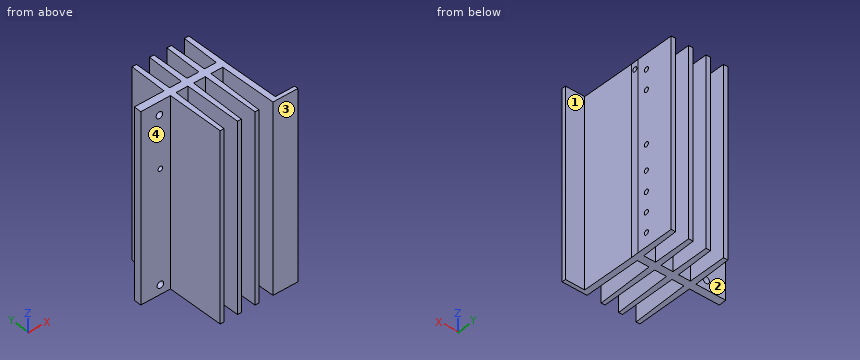
```python
from build123d import *

# Parameters (mm, degrees)
SKICA1_W                 = 93
SKICA1_H                 = 4
P_IDAT_VYSUNUT_M1_DEPTH  = 100
SKICA2_W                 = 121.490565888
SKICA2_H                 = 20.366839506
ODEBRAT_VYSUNUT_M1_DEPTH = 204.75436619
SKICA3_W                 = 67.97848113
SKICA3_H                 = 83.569638829
ODEBRAT_VYSUNUT_M2_DEPTH = 198.590610741
SKICA4_R                 = 1.25
ODEBRAT_VYSUNUT_M3_DEPTH = 5
SKICA5_R                 = 1.25
ODEBRAT_VYSUNUT_M4_DEPTH = 16
SKICA6_R                 = 1.25
ODEBRAT_VYSUNUT_M5_DEPTH = 5
SKICA7_R                 = 1.75
ODEBRAT_VYSUNUT_M6_DEPTH = 10


with BuildPart() as part:
    # Skica1 → Přidat vysunutím1 (new body)
    with BuildSketch(Plane.XY):
        Polygon((83.039921415, 64.689614429), (83.539921415, 94.689614429), (80.539921415, 94.689614429), (81.039921415, 64.689614429), align=None)
        Polygon((92.289921415, 64.689614429), (92.789921415, 94.689614429), (89.789921415, 94.689614429), (90.289921415, 64.689614429), align=None)
        Polygon((101.539921415, 64.689614429), (102.039921415, 94.689614429), (99.039921415, 94.689614429), (99.539921415, 64.689614429), align=None)
        Polygon((112.011784527, 66.689614429), (111.289921415, 94.689614429), (108.281882654, 94.689614429), (109.055307417, 64.689614429), (122.289921415, 64.689614429), (122.289921415, 66.689614429), align=None)
        Polygon((108.289921415, 98.689614429), (111.289921415, 98.689614429), (110.789921415, 128.689614429), (108.789921415, 128.689614429), align=None)
        Polygon((99.039921415, 98.689614429), (102.039921415, 98.689614429), (101.539921415, 128.689614429), (99.539921415, 128.689614429), align=None)
        Polygon((89.789921415, 98.689614429), (92.789921415, 98.689614429), (92.289921415, 128.689614429), (90.289921415, 128.689614429), align=None)
        Polygon((80.539921415, 98.689614429), (83.539921415, 98.689614429), (83.039921415, 128.689614429), (81.039921415, 128.689614429), align=None)
        with Locations((64.789921415, 96.689614429)):
            Rectangle(SKICA1_W, SKICA1_H)
        Polygon((27.539921415, 98.689614429), (30.539921415, 98.689614429), (30.039921415, 128.689614429), (28.039921415, 128.689614429), align=None)
        Polygon((36.789921415, 98.689614429), (39.789921415, 98.689614429), (39.289921415, 128.689614429), (37.289921415, 128.689614429), align=None)
        Polygon((46.039921415, 98.689614429), (49.039921415, 98.689614429), (48.539921415, 128.689614429), (46.539921415, 128.689614429), align=None)
        Polygon((18.289921415, 98.689614429), (21.289921415, 98.689614429), (20.789921415, 128.689614429), (18.789921415, 128.689614429), align=None)
        Polygon((20.524535413, 64.689614429), (21.297960175, 94.689614429), (18.289921415, 94.689614429), (17.568058303, 66.689614429), (7.289921415, 66.689614429), (7.289921415, 64.689614429), align=None)
        Polygon((30.039921415, 64.689614429), (30.539921415, 94.689614429), (27.539921415, 94.689614429), (28.039921415, 64.689614429), align=None)
        Polygon((39.289921415, 64.689614429), (39.789921415, 94.689614429), (36.789921415, 94.689614429), (37.289921415, 64.689614429), align=None)
        Polygon((48.539921415, 64.689614429), (49.039921415, 94.689614429), (46.039921415, 94.689614429), (46.539921415, 64.689614429), align=None)
    extrude(amount=P_IDAT_VYSUNUT_M1_DEPTH)

    # Skica2 → Odebrat vysunutím1 (cut, through all)
    with BuildSketch(Plane.XY.offset(100)):
        with Locations((69.111954217, 128.873034182)):
            Rectangle(SKICA2_W, SKICA2_H)
    extrude(amount=-ODEBRAT_VYSUNUT_M1_DEPTH, mode=Mode.SUBTRACT)

    # Skica3 → Odebrat vysunutím2 (cut, through all)
    with BuildSketch(Plane.XY.offset(100)):
        with Locations((30.80068085, 79.614929898)):
            Rectangle(SKICA3_W, SKICA3_H)
    extrude(amount=-ODEBRAT_VYSUNUT_M2_DEPTH, mode=Mode.SUBTRACT)

    # Skica4 → Odebrat vysunutím3 (cut)
    with BuildSketch(Plane(origin=(111.289921415, 0, 0), x_dir=(0, 0, -1), z_dir=(1, 0, 0))):
        with Locations(Location((-91.74, 103.689614429, 0), (0, 0, 90))):
            Circle(SKICA4_R)
        with Locations(Location((-81.24, 103.689614429, 0), (0, 0, 90))):
            Circle(SKICA4_R)
        with Locations(Location((-53.01, 103.689614429, 0), (0, 0, 90))):
            Circle(SKICA4_R)
        with Locations(Location((-28.47, 103.689614429, 0), (0, 0, 90))):
            Circle(SKICA4_R)
        with Locations(Location((-17.97, 103.689614429, 0), (0, 0, 90))):
            Circle(SKICA4_R)
        with Locations(Location((-7.43, 103.689614429, 0), (0, 0, 90))):
            Circle(SKICA4_R)
        with Locations(Location((-39.47, 103.689614429, 0), (0, 0, 90))):
            Circle(SKICA4_R)
    extrude(amount=-ODEBRAT_VYSUNUT_M3_DEPTH, mode=Mode.SUBTRACT)

    # Skica5 → Odebrat vysunutím4 (cut)
    with BuildSketch(Plane(origin=(111.289921415, 0, 0), x_dir=(0, 0, -1), z_dir=(1, 0, 0))):
        with Locations((-96, 96.689614429)):
            Circle(SKICA5_R)
    extrude(amount=-ODEBRAT_VYSUNUT_M4_DEPTH, mode=Mode.SUBTRACT)

    # Skica6 → Odebrat vysunutím5 (cut)
    with BuildSketch(Plane.XZ.offset(-94.689614429)):
        with Locations((74.677082764, 93)):
            Circle(SKICA6_R)
        with Locations((75.177082764, 5)):
            Circle(SKICA6_R)
        with Locations((75.177082764, 65)):
            Circle(SKICA6_R)
    extrude(amount=-ODEBRAT_VYSUNUT_M5_DEPTH, mode=Mode.SUBTRACT)

    # Skica7 → Odebrat vysunutím6 (cut)
    with BuildSketch(Plane.XZ.offset(-94.689614429)):
        with Locations((75.177082764, 5)):
            Circle(SKICA7_R)
        with Locations((74.677082764, 93)):
            Circle(SKICA7_R)
    extrude(amount=-ODEBRAT_VYSUNUT_M6_DEPTH, mode=Mode.SUBTRACT)


solid = part.part
```
Source: CAD feature listing. Evaluate the final solid. Frame: model axes, mm. Face numbers are marked on the shaded views. A direction names the side the tool comes from. Round coordinates to 2 decimals unless told otherwise and drop trailing zeros. Write each loop counter-clockwise with the first axis right and the second up, starting at its lowest first coordinate (ties: lowest second). Pieces come first, ordered by that corner, then holes. Notation, with made-up numbers: M -27.75,-2.5 L 5.25,-2.5 A11 ccw 5.25,4.5 Z; hole C 34.5,-17.75 d3. An arc over 180 degrees is marked long. Answer as a JSON object with one key per item and string values. Group by question number.
(1) Ray query, line 1 (X direction, y = 96, z = 65); line 2 (X direction, y = 74, z = 88); line 3 (X direction, y = 91, z = 83). Return the intervals inside material, ascending. Write a range as [from, to].
(2) Reachability of the marked faces 1, 2, 3 and 4 from +Z, -Z, +X, -X, +Y, -Y: full face, straight path, thin tool, end or side. Return the list, or none.
(3) Section query A-A on y = 80.5. Output: boundary loops of the cut face in (x, z).
(4) Section query D-D on y = 110. Output: boundary loops of the cut face in (x, z), then the cut area to 3 significant figures.
(5) Section query C-C on x = 115. Output: boundary loops of the cut face in (y, z).
(6) Section query B-B on x = 105. Output: boundary loops of the cut face in (y, z).
(7) First-contact query: pin 1 (2 mm diameter, centred on x = 75.18, z = 5, fed in from +Y); pin 2 (5 mm diameter, centred on x = 105.5, z = 46, fed in from -Y); pin 3 (1.5 mm diameter, centred on x = 96, z = 27, fed in from +Y); pin 4 (10 mm diameter, centred on x = 82.5, y = 111.5, fed in from -Z). Flat tips, straight axial feed; report the tip coordinate or a pass-through.
Computed values:
{
 "1": {"line 1": "[64.79, 73.93], [76.43, 111.29]", "line 2": "[80.88, 83.2], [90.13, 92.45], [99.38, 101.7], [108.82, 111.82]", "line 3": "[80.6, 83.48], [89.85, 92.73], [99.1, 101.98], [108.38, 111.39]"},
 "2": {"face 1": "+Z, -Z, +X, +Y", "face 2": "+Z, -Z, -X, +Y", "face 3": "+Z, -Z, +X, -X, -Y", "face 4": "+Z, -Z, -X, -Y"},
 "3": {"outline": "M 80.78,0 L 83.3,0 L 83.3,100 L 80.78,100 Z; M 90.03,0 L 92.55,0 L 92.55,100 L 90.03,100 Z; M 99.28,0 L 101.8,0 L 101.8,100 L 99.28,100 Z; M 108.65,0 L 111.66,0 L 111.66,100 L 108.65,100 Z"},
 "4": {"outline": "M 80.73,0 L 83.35,0 L 83.35,100 L 80.73,100 Z; M 89.98,0 L 92.6,0 L 92.6,100 L 89.98,100 Z; M 99.23,0 L 101.85,0 L 101.85,100 L 99.23,100 Z; M 108.48,0 L 111.1,0 L 111.1,100 L 108.48,100 Z", "area": "1,050 mm^2"},
 "5": {"outline": "M 64.69,0 L 66.69,0 L 66.69,100 L 64.69,100 Z"},
 "6": {"outline": "M 94.69,0 L 98.69,0 L 98.69,100 L 94.69,100 Z; hole C 96.69,96 d2.5"},
 "7": {"pin 1": "through", "pin 2": "y = 94.69", "pin 3": "y = 98.69", "pin 4": "z = 0"}
}
